```python
from build123d import *

# Parameters (mm, degrees)
BOSS_EXTRUDE1_DEPTH = 13
BOSS_EXTRUDE2_DEPTH = 3.5


with BuildPart() as part:
    # Sketch1 → Boss-Extrude1 (new body)
    with BuildSketch(Plane(origin=(0, 0, 0), x_dir=(1, 0, 0), z_dir=(0, 1, 0))):
        with BuildLine():
            Line((-70.343588137, -14.533254602), (-55.810333535, 0))
            Line((-55.810333535, 0), (-46.739265723, 0))
            Line((-46.739265723, 0), (-46.739265723, -5))
            Line((-46.739265723, -5), (-53.739265723, -5))
            Line((-53.739265723, -5), (-65.02750007, -16.288234347))
            ThreePointArc((-65.02750007, -16.288234347), (8.153517743, -70.494428377), (65.810333535, 0))
            Line((65.810333535, 0), (77.98664195, 0))
            Line((77.98664195, 0), (77.98664195, -5))
            Line((77.98664195, -5), (70.98664195, -5))
            ThreePointArc((70.98664195, -5), (4.777459092, -75.825696043), (-70.343588137, -14.533254602))
        make_face()
    extrude(amount=BOSS_EXTRUDE1_DEPTH)

    # Sketch2 → Boss-Extrude2 (add)
    with BuildSketch(Plane.XZ):
        with BuildLine():
            Line((-65.02750007, 16.288234347), (-68.563033976, 12.752700441))
            Line((-68.563033976, 12.752700441), (-70.343588137, 14.533254602))
            ThreePointArc((-70.343588137, 14.533254602), (7.270373797, 75.613348598), (70.810333535, 0))
            Line((70.810333535, 0), (65.810333535, 0))
            ThreePointArc((65.810333535, 0), (8.153517743, 70.494428377), (-65.02750007, 16.288234347))
        make_face()
    extrude(amount=BOSS_EXTRUDE2_DEPTH)


solid = part.part
```
For this review, take the finished solid that the model builds, in its own axes (mm). A direction names the side the tool comes from. Round coordinates to 2 decimals unless told otherwise and drop trailing zeros. Write each loop counter-clockwise with the first axis right and the second up, starting at its lowest first coordinate (ties: lowest second). Pieces come first, ordered by that corner, then holes. Notation, with made-up numbers: (37.25, 36.5) - (65.25, 36.5) arc R5 ccw to (65.25, 41.5) - close; hole circle Ø7 at (8, 20). An arc over 180 degrees is marked (long way). Answer as CSV lines item,"result". Start each with the question number.
(1) Add section A-A, the plane z = 60.5. State the section outline as (x, y) points, plus the area to 3 significant figures.
(2) Add section D-D, the plane z = 51.5. State the section outline as (x, y) points.
(3) For line 1 (Z direction, x = -57, y = 7); line 2 (X direction, y = 4.5, z = 47); line 3 (X direction, y = 4.5, z = 32.5), list the stretches that pass through material, from the lowest coordinate up.
(4) Mouldability with a two-part tool opening along Z and no side actions: class faces 5 (the cylindrical face through (9.548, 4.866, 70.306)), 6 (the flat face through (1, -3.5, 72)), 7 (the flat face through (75, 6, 5)), 8 (the flat face through (-51, 6, 0)) as +Z half, -Z half, draft (parallel to the pull), parting line (faces both ways), or undercut.
(5) Add section C-C, the plane x = 0. State the section outline as (y, z) points.
(6) For pin 1 (1.5 mm diameter, centred on x = 74, z = 3, fed in from -Y); pin 2 (2 mm diameter, centred on x = -50, y = 4.5, fed in from +Z); pin 3 (8 mm diameter, centred on y = 1.5, z = 25.5, fed in from -X), all flat-tipped, find the tip position at first contact; note any pin that passes through.
(7) Machinability: for faces 1 (the flat face through (77.987, 6, 2)), 2 (the flat face through (-46.739, 6, 2)), 3 (the flat face through (-66.771, -1.726, 14.545)), 4 (the flat face through (-59.304, 6.409, 10.565)), which of the approach directions +Z, -Z, +X, -X, +Y, -Y give a long, thin tool a straight path to every point of the face, cutting with its end or side? Answer none if there is none.
From the geometry:
1,outline,"(-44.26, -3.5) - (-35.72, -3.5) - (-35.72, 13) - (-44.26, 13) - close; (35.72, -3.5) - (44.26, -3.5) - (44.26, 13) - (35.72, 13) - close"
1,area,"282 mm²"
2,outline,"(-53.64, -3.5) - (-46.84, -3.5) - (-46.84, 13) - (-53.64, 13) - close; (46.84, -3.5) - (53.64, -3.5) - (53.64, 13) - (46.84, 13) - close"
3,line 1,"z = 1.19 to 8.26, 38.27 to 47.31"
3,line 2,"x = -57.23 to -50.91, 50.91 to 57.23"
3,line 3,"x = -65.44 to -60, 60 to 65.44"
4,face 5,"undercut"
4,face 6,"draft"
4,face 7,"+Z half"
4,face 8,"-Z half"
5,outline,"(-3.5, 71) - (13, 71) - (13, 75.99) - (-3.5, 75.99) - close"
6,pin 1,"stops at y = 0"
6,pin 2,"stops at z = 56.36"
6,pin 3,"stops at x = -69.04"
7,face 1,"+Z, -Z, +X, +Y, -Y"
7,face 2,"-Z, +Y, -Y"
7,face 3,"-Z, -Y"
7,face 4,"+Y, -Y"
